Verification items for the finished model (mm, model axes). Face numbers are marked on the shaded views. A direction names the side the tool comes from. Round coordinates to 2 decimals unless told otherwise and drop trailing zeros. Write each loop counter-clockwise with the first axis right and the second up, starting at its lowest first coordinate (ties: lowest second). Pieces come first, ordered by that corner, then holes.
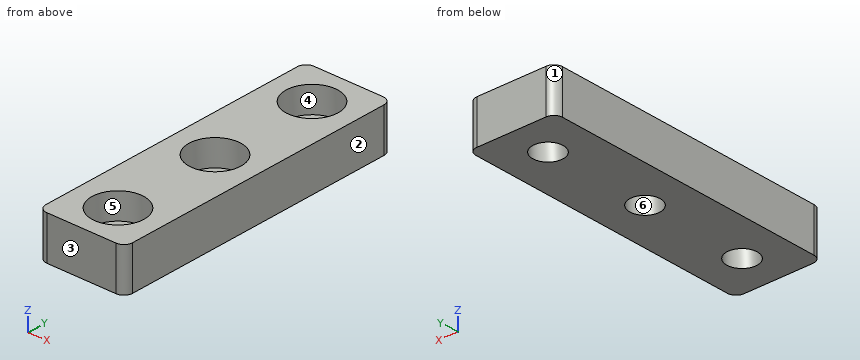
from build123d import *

# Parameters (mm, degrees)
SKETCH1_W           = 10
SKETCH1_H           = 34.4
BOSS_EXTRUDE1_DEPTH = 5
FILLET1_R           = 1
SKETCH4_R           = 1.75
CUT_EXTRUDE1_DEPTH  = 5
SKETCH5_R           = 3
CUT_EXTRUDE2_DEPTH  = 3


with BuildPart() as part:
    # Sketch1 → Boss-Extrude1 (new body)
    with BuildSketch(Plane.XY):
        Rectangle(SKETCH1_W, SKETCH1_H)
    extrude(amount=BOSS_EXTRUDE1_DEPTH)

    # Fillet1
    fillet1_edges = [part.edges().sort_by_distance(p)[0] for p in [
        (-5, 17.2, 2.5),
        (5, 17.2, 2.5),
        (5, -17.2, 2.5),
        (-5, -17.2, 2.5),
    ]]
    fillet(fillet1_edges, radius=FILLET1_R)

    # Sketch4 → Cut-Extrude1 (cut)
    with BuildSketch(Plane.XY.offset(5)):
        Circle(SKETCH4_R)
        with Locations((0, 12.5)):
            Circle(SKETCH4_R)
        with Locations((0, -12.5)):
            Circle(SKETCH4_R)
    extrude(amount=-CUT_EXTRUDE1_DEPTH, mode=Mode.SUBTRACT)

    # Sketch5 → Cut-Extrude2 (cut)
    with BuildSketch(Plane.XY.offset(5)):
        with Locations((0, 12.5)):
            Circle(SKETCH5_R)
        Circle(SKETCH5_R)
        with Locations((0, -12.5)):
            Circle(SKETCH5_R)
    extrude(amount=-CUT_EXTRUDE2_DEPTH, mode=Mode.SUBTRACT)


solid = part.part
Q1. Sectioned sample at A-A (x = 0). Enter the section's corners in (y, z), plus the area to 3 significant figures.
Recorded:
outline: (-17.2, 0) - (-14.25, 0) - (-14.25, 2) - (-15.5, 2) - (-15.5, 5) - (-17.2, 5) - close; (-10.75, 0) - (-1.75, 0) - (-1.75, 2) - (-3, 2) - (-3, 5) - (-9.5, 5) - (-9.5, 2) - (-10.75, 2) - close; (1.75, 0) - (10.75, 0) - (10.75, 2) - (9.5, 2) - (9.5, 5) - (3, 5) - (3, 2) - (1.75, 2) - close; (14.25, 0) - (17.2, 0) - (17.2, 5) - (15.5, 5) - (15.5, 2) - (14.25, 2) - close
area: 97.0 mm2
Q2. Depth check by flat-ended pin: P1, Ø4.5, axis at x = 0, y = 0, coming from the +Z side; P2, Ø1.8, axis at x = -0.5, y = -12.5, coming from the +Z side. Enter the tip coordinate at first touch or a pass-through.
Recorded:
P1: stops at z = 2
P2: passes through
Q3. Sectioned sample at B-B (z = 1). Enter the section's corners in (x, y).
Recorded:
outline: (-5, -16.2) arc R1 ccw to (-4, -17.2) - (4, -17.2) arc R1 ccw to (5, -16.2) - (5, 16.2) arc R1 ccw to (4, 17.2) - (-4, 17.2) arc R1 ccw to (-5, 16.2) - close; hole circle Ø3.5 at (0, -12.5); hole circle Ø3.5 at (0, 0); hole circle Ø3.5 at (0, 12.5)
Q4. Tool access check on the marked faces 5 and 6. Record the directions out of +Z, -Z, +X, -X, +Y, -Y that give a thin tool (end or side, any length) a straight path to the whole face; none if there is none.
Recorded:
face 5: +Z
face 6: +Z, -Z
Q5. Sectioned sample at D-D (x = 2.5). Enter the section's corners in (y, z), plus the area to 3 significant figures.
Recorded:
outline: (-17.2, 0) - (17.2, 0) - (17.2, 5) - (14.16, 5) - (14.16, 2) - (10.84, 2) - (10.84, 5) - (1.66, 5) - (1.66, 2) - (-1.66, 2) - (-1.66, 5) - (-10.84, 5) - (-10.84, 2) - (-14.16, 2) - (-14.16, 5) - (-17.2, 5) - close
area: 142 mm2
Q6. Material ranges on line 1 along Y through (x, z) = (0, 0.75); line 2 along Y through (x, z) = (0, 3.1); line 3 along Z through (x, y) = (-0.5, 2), recorded low to high.
Recorded:
line 1: y = -17.2 to -14.25, -10.75 to -1.75, 1.75 to 10.75, 14.25 to 17.2
line 2: y = -17.2 to -15.5, -9.5 to -3, 3 to 9.5, 15.5 to 17.2
line 3: z = 0 to 2
Q7. Sectioned sample at C-C (y = 13.5). Enter the section's corners in (x, z).
Recorded:
outline: (-5, 0) - (-1.44, 0) - (-1.44, 2) - (-2.83, 2) - (-2.83, 5) - (-5, 5) - close; (1.44, 0) - (5, 0) - (5, 5) - (2.83, 5) - (2.83, 2) - (1.44, 2) - close
Q8. Release check for a two-part mould opening along X. For the marked faces 1, 2, 3 and 4 record: released by +X, released by -X, zero draft, split by the parting line, or undercut.
Recorded:
face 1: released by -X
face 2: released by +X
face 3: zero draft
face 4: undercut
